Autodesk Inventor part; units mm, degrees
ref_plane "YZ Plane" through (0, 0, 0) normal (1, 0, 0) x (0, 1, 0)
ref_plane "XZ Plane" through (0, 0, 0) normal (0, 1, 0) x (-1, 0, 0)
ref_plane "XY Plane" through (0, 0, 0) normal (0, 0, 1) x (1, 0, 0)
ref_plane "Work Plane2" through (0, 1, 0) normal (0, 1, 0) x (1, 0, 0)
sketch "Sketch2" plane through (0, 1, 0) normal (0, 1, 0) x (1, 0, 0)
  arc A0 (-13.8229, -33.4026) -> (-9.8229, -37.4026) centre (-9.8229, -33.4026) ccw
  arc A1 (-9.8229, 36.9551) -> (-13.8229, 32.9551) centre (-9.8229, 32.9551) ccw
  circle A2 centre (2.4699, 39.3408) radius 1.55
  circle A3 centre (26.9336, -22.3933) radius 1.55
  circle A4 centre (-9.8229, -33.4026) radius 1.55
  line L0 (23.7927, 44.0538) -> (31.7927, 44.0538)
  line L1 (32.7927, 43.0538) -> (32.7927, 26.8418)
  line L2 (29.7927, 23.8418) -> (25.2541, 23.8418)
  line L3 (-17.8229, 3.7762) -> (-42.9549, 3.7762)
  line L4 (-43.9549, 2.7762) -> (-43.9549, -3.2238)
  line L5 (-42.9549, -4.2238) -> (-17.8229, -4.2238)
  line L6 (28.7927, -43.9467) -> (31.7927, -43.9467)
  line L7 (22.7927, 43.0538) -> (22.7927, 42.5538)
  arc A5 (23.7927, 44.0538) -> (22.7927, 43.0538) centre (23.7927, 43.0538) ccw
  arc A6 (32.7927, 43.0538) -> (31.7927, 44.0538) centre (31.7927, 43.0538) ccw
  arc A7 (31.7927, -43.9467) -> (32.7927, -42.9467) centre (31.7927, -42.9467) ccw
  arc A8 (27.7927, -42.9467) -> (28.7927, -43.9467) centre (28.7927, -42.9467) ccw
  arc A9 (29.7927, 23.8418) -> (32.7927, 26.8418) centre (29.7927, 26.8418) ccw
  arc A10 (19.7927, 39.5538) -> (22.7927, 42.5538) centre (19.7927, 42.5538) ccw
  arc A11 (-42.9549, 3.7762) -> (-43.9549, 2.7762) centre (-42.9549, 2.7762) ccw
  arc A12 (-43.9549, -3.2238) -> (-42.9549, -4.2238) centre (-42.9549, -3.2238) ccw
  line L8 (-13.8229, 32.9551) -> (-13.8229, 19.9551)
  line L9 (-14.8229, 18.9551) -> (-15.8229, 18.9551)
  line L10 (-16.8229, 17.9551) -> (-16.8229, 4.7762)
  line L11 (-13.8229, -33.4026) -> (-13.8229, -20.4026)
  line L12 (-14.8229, -19.4026) -> (-15.8229, -19.4026)
  line L13 (-16.8229, -18.4026) -> (-16.8229, -5.2238)
  arc A13 (-14.8229, 18.9551) -> (-13.8229, 19.9551) centre (-14.8229, 19.9551) ccw
  arc A14 (-15.8229, 18.9551) -> (-16.8229, 17.9551) centre (-15.8229, 17.9551) ccw
  arc A15 (-17.8229, 3.7762) -> (-16.8229, 4.7762) centre (-17.8229, 4.7762) ccw
  arc A16 (-16.8229, -5.2238) -> (-17.8229, -4.2238) centre (-17.8229, -5.2238) ccw
  arc A17 (-16.8229, -18.4026) -> (-15.8229, -19.4026) centre (-15.8229, -18.4026) ccw
  arc A18 (-13.8229, -20.4026) -> (-14.8229, -19.4026) centre (-14.8229, -20.4026) ccw
  arc A19 (2.4699, 43.3408) -> (-1.5298, 39.3918) centre (2.4699, 39.3408) ccw
  line L14 (-1.5298, 39.3918) -> (-1.5298, 36.9551)
  line L15 (-1.5298, 36.9551) -> (-9.8229, 36.9551)
  line L16 (12.2983, -43.9467) -> (1.2983, -43.9467)
  line L17 (0.2983, -42.9467) -> (0.2983, -38.4026)
  line L18 (-0.7017, -37.4026) -> (-9.8229, -37.4026)
  arc A20 (0.2983, -42.9467) -> (1.2983, -43.9467) centre (1.2983, -42.9467) ccw
  arc A21 (12.2983, -43.9467) -> (13.2983, -42.9467) centre (12.2983, -42.9467) ccw
  arc A22 (0.2983, -38.4026) -> (-0.7017, -37.4026) centre (-0.7017, -38.4026) ccw
  line L19 (19.7927, 39.5538) -> (8.4489, 39.5538)
  line L20 (27.7927, -42.9467) -> (27.7927, -40.9467)
  line L21 (25.7927, -38.9467) -> (15.2983, -38.9467)
  arc A23 (27.7927, -40.9467) -> (25.7927, -38.9467) centre (25.7927, -40.9467) ccw
  line L22 (13.2983, -42.9467) -> (13.2983, -40.9467)
  arc A24 (15.2983, -38.9467) -> (13.2983, -40.9467) centre (15.2983, -40.9467) ccw
  line L23 (8.4489, 39.5538) -> (6.4642, 39.5538)
  arc A25 (6.4642, 39.5538) -> (2.4699, 43.3408) centre (2.4699, 39.3408) ccw
  line L24 (25.2541, -19.1582) -> (28.7927, -19.1582)
  line L25 (28.7927, -19.1582) -> (28.7927, -19.1582)
  line L26 (29.7927, -20.1582) -> (29.7927, -29.8512)
  line L27 (32.7927, -42.9467) -> (32.7927, -31.8512)
  line L28 (31.7927, -30.8512) -> (30.7927, -30.8512)
  arc A26 (29.7927, -20.1582) -> (28.7927, -19.1582) centre (28.7927, -20.1582) ccw
  arc A27 (29.7927, -29.8512) -> (30.7927, -30.8512) centre (30.7927, -29.8512) ccw
  arc A28 (32.7927, -31.8512) -> (31.7927, -30.8512) centre (31.7927, -31.8512) ccw
  line L29 (25.2541, 23.8418) -> (23.8455, 23.8418)
  line L30 (21.9025, 21.3673) -> (25.9693, 4.7141)
  line L31 (25.9693, -0.0306) -> (21.9025, -16.6838)
  line L32 (23.8455, -19.1582) -> (25.7927, -19.1582)
  arc A29 (23.8455, 23.8418) -> (21.9025, 21.3673) centre (23.8455, 21.8418) ccw
  arc A30 (21.9025, -16.6838) -> (23.8455, -19.1582) centre (23.8455, -17.1582) ccw
  arc A31 (25.9693, -0.0306) -> (25.9693, 4.7141) centre (16.2548, 2.3418) ccw
  point P0 (0, 0)
  point P1 (22.7927, 44.0538)
  point P2 (32.7927, 44.0538)
  point P3 (32.7927, 23.8418)
  point P4 (32.7927, -43.9467)
  point P5 (-16.8229, 3.7762)
  point P6 (-16.8229, -4.2238)
  point P7 (21.2983, 23.8418)
  point P8 (30.2927, -43.9467)
  point P9 (-13.8229, 18.9551)
  point P10 (-16.8229, 18.9551)
  point P11 (-13.8229, -19.4026)
  point P12 (-16.8229, -19.4026)
  point P13 (13.2983, -43.9467)
  point P14 (0.2983, -43.9467)
  point P15 (0.2983, -37.4026)
  point P16 (27.7927, -38.9467)
  point P17 (27.7927, -42.9467)
  point P18 (29.7927, -19.1582)
  point P19 (27.0234, -19.1582)
  point P20 (27.5234, 23.8418)
  point P21 (26.5486, 2.3418)
  dimension "d13" = 3.1
  dimension "d15" = 3.1
  dimension "d26" = 1
  dimension "d27" = 3
  dimension "d32" = 1
  dimension "d33" = 20.212
  dimension "d36" = 14
  dimension "d37" = 3
  dimension "d38" = 14
  dimension "d39" = 3
  dimension "d40" = 1
  dimension "d42" = 13
  dimension "d43" = 1
  dimension "d47" = 88.0005
  dimension "d49" = 4
  dimension "d50" = 2
  dimension "d51" = 2
  dimension "d52" = 0.5
  dimension "d57" = 1
  dimension "d58" = 43
  dimension "d60" = 21.5
  dimension "d61" = 2
  dimension "d62" = 10
extrude "Extrusion2" add sketch "Sketch2" along normal blind 1
properties part number "pcb"
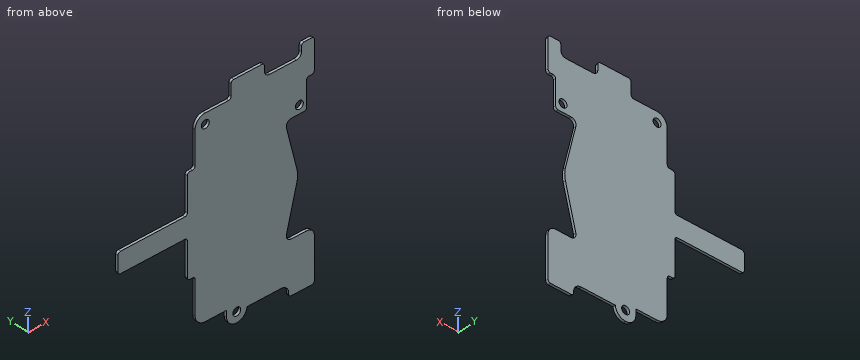
Part model, mm, in its own coordinate system. Give positions to 0.01 mm unless a question says otherwise; leave off trailing zeros. Order: outer loops, then holes, each group sorted by start corner. A loop starts at its lowest first (then second) coordinate and runs counter-clockwise, first axis right, second up. Notation, with made-up numbers: M -28,70 L -17,70 A19 ccw -17,92 Z; hole C 12,48.25 d11. An arc over 180 degrees is marked long. Use a Markdown table: item, result. Add a question column.
(1) Saw through at B-B, the plane z = 13. Give the cut face in (x, y), and give its area (3 significant figures).
(2) Probe line 1 along X through (y, z) = (1.9, 22.5); line 2 along Z through (x, y) = (2.5, 1.7); line 3 along Z through (x, y) = (-23, 1.5). List the from-to ranges inside material, lowest first. Write a range as [from, to].
(3) Drop flat-ended pins along their axis: P1, Ø0.5, axis at x = 15, y = 1.5, coming from the -Z side; P2, Ø3, axis at x = 2.47, z = -39.34, coming from the +Y side. Give the stop position or say it passes through.
(4) Saw through at A-A, the plane x = -25.5. Give the cut face in (y, z).
(5) Saw through at C-C, the plane y = 1.45. Give the number of separate pieces and of enclosed holes in the cut face, and give its area (3 significant figures).
Answer key:
| question | item | result |
|---|---|---|
| 1 | outline | M -16.82,1 L 22.8,1 L 22.8,2 L -16.82,2 Z |
| 1 | area | 39.6 mm^2 |
| 2 | line 1 | [-13.82, 25.39], [28.48, 29.79] |
| 2 | line 2 | [-43.34, -40.89], [-37.79, 43.95] |
| 2 | line 3 | [-3.78, 4.22] |
| 3 | P1 | z = -39.55 |
| 3 | P2 | through |
| 4 | outline | M 1,-3.78 L 2,-3.78 L 2,4.22 L 1,4.22 Z |
| 5 | separate pieces | 1 |
| 5 | enclosed holes | 3 |
| 5 | area | 3,650 mm^2 |
